Design review of the part built by this model. Coordinates are the model's own, in mm. Face numbers are marked on the shaded views. A direction names the side the tool comes from. Coordinates: 2 decimals unless noted, no trailing zeros. Order: outer loops, then holes, each group sorted by start corner. A loop starts at its lowest first (then second) coordinate and runs counter-clockwise, first axis right, second up. Notation, with made-up numbers: M -11.75,-31.75 L 30.25,-31.75 A17 cw 30.25,-6.75 Z; hole C -13,-12.75 d8. An arc over 180 degrees is marked long. Answer as a JSON object with one key per item and string values.
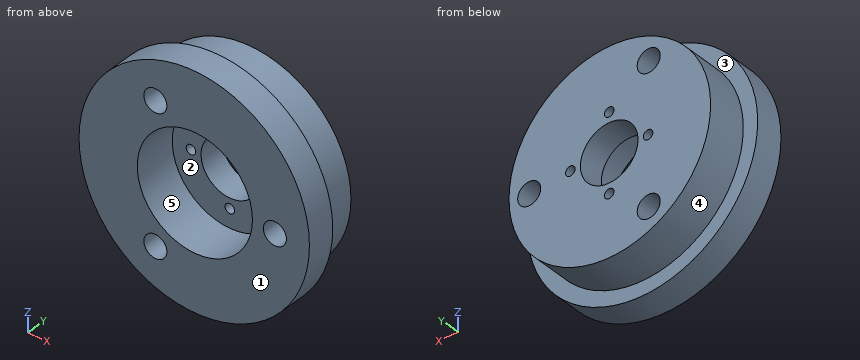
from build123d import *

# Parameters (mm, degrees)
SKETCH2_R               = 10
SKETCH2_R_2             = 1.65
CUT_EXTRUDE2_DEPTH      = 1
CUT_EXTRUDE2_DEPTH_BACK = 25
SKETCH2_5_R             = 20
SKETCH2_5_R_2           = 1.65
SKETCH2_5_R_3           = 10
CUT_EXTRUDE3_DEPTH      = 15
SKETCH3_R               = 4
CUT_EXTRUDE4_DEPTH      = 1
CUT_EXTRUDE4_DEPTH_BACK = 25


with BuildPart() as part:
    # Sketch1 → Revolve1 (revolve)
    with BuildSketch(Plane.XY):
        Polygon((-40, 10), (-35, 10), (-35, 24), (0, 24), (0, 0), (-40, 0), align=None)
    revolve(axis=Axis((0, -1000, 0), (0, 1, 0)))

    # Sketch2 → Cut-Extrude2 (cut, two sides)
    with BuildSketch(Plane.XZ) as cut_extrude2_sk:
        with Locations((0.220332098, -0.275415123)):
            Circle(SKETCH2_R)
        with Locations((13.720332098, -0.275415123)):
            Circle(SKETCH2_R_2)
        with Locations((0.220332098, -13.775415123)):
            Circle(SKETCH2_R_2)
        with Locations((-13.279667902, -0.275415123)):
            Circle(SKETCH2_R_2)
        with Locations((0.220332098, 13.224584877)):
            Circle(SKETCH2_R_2)
    extrude(amount=CUT_EXTRUDE2_DEPTH, mode=Mode.SUBTRACT)
    extrude(cut_extrude2_sk.sketch, amount=-CUT_EXTRUDE2_DEPTH_BACK, mode=Mode.SUBTRACT)

    # Sketch2<5> → Cut-Extrude3 (cut)
    with BuildSketch(Plane.XZ):
        with Locations((0.220332098, -0.275415123)):
            Circle(SKETCH2_5_R)
        with Locations((0.220332098, -13.775415123)):
            Circle(SKETCH2_5_R_2, mode=Mode.SUBTRACT)
        with Locations((13.720332098, -0.275415123)):
            Circle(SKETCH2_5_R_2, mode=Mode.SUBTRACT)
        with Locations((0.220332098, -0.275415123)):
            Circle(SKETCH2_5_R_3, mode=Mode.SUBTRACT)
        with Locations((-13.279667902, -0.275415123)):
            Circle(SKETCH2_5_R_2, mode=Mode.SUBTRACT)
        with Locations((0.220332098, 13.224584877)):
            Circle(SKETCH2_5_R_2, mode=Mode.SUBTRACT)
    extrude(amount=-CUT_EXTRUDE3_DEPTH, mode=Mode.SUBTRACT)

    # Sketch3 → Cut-Extrude4 (cut, two sides)
    with BuildSketch(Plane(origin=(0, 24, 0), x_dir=(1, 0, 0), z_dir=(0, 1, 0))) as cut_extrude4_sk:
        with Locations((28, 1.382050236)):
            Circle(SKETCH3_R)
        with Locations((-13.5, -24.11)):
            Circle(SKETCH3_R)
        with Locations((-13.5, 24.11473671)):
            Circle(SKETCH3_R)
    extrude(amount=CUT_EXTRUDE4_DEPTH, mode=Mode.SUBTRACT)
    extrude(cut_extrude4_sk.sketch, amount=-CUT_EXTRUDE4_DEPTH_BACK, mode=Mode.SUBTRACT)


solid = part.part
1) Tool access review of the marked faces 1 and 2: name each direction out of +Z, -Z, +X, -X, +Y, -Y from which nothing blocks a thin tool from reaching the whole face with its end or side.
Taken from the geometry:
{"face 1": "+Z, -Z, +X, -X, -Y", "face 2": "-Y"}
2) Add section D-D (x = 21.5). State the section outline as (y, z) points, and give its area (3 significant figures).
Taken from the geometry:
{"outline": "M 0,-33.73 L 10,-33.73 L 10,-27.62 L 24,-27.62 L 24,27.62 L 10,27.62 L 10,33.73 L 0,33.73 Z", "area": "1,450 mm2"}
3) Add section C-C (y = 17.25). Count the separate pieces of the cut face and the enclosed holes in it, and give its area (3 significant figures).
Taken from the geometry:
{"separate pieces": "1", "enclosed holes": "8", "area": "3,350 mm2"}
4) Add section A-A (z = 27). State the section outline as (x, y) points, and give its area (3 significant figures).
Taken from the geometry:
{"outline": "M -29.51,0 L -16.27,0 L -16.27,24 L -22.27,24 L -22.27,10 L -29.51,10 Z; M -10.73,0 L 29.51,0 L 29.51,10 L 22.27,10 L 22.27,24 L -10.73,24 Z", "area": "1,080 mm2"}
5) Mouldability with a two-part tool opening along X and no side actions: class the marked faces 3, 4 and 5 as released by +X, released by -X, zero draft, split by the parting line, or undercut.
Taken from the geometry:
{"face 3": "zero draft", "face 4": "split by the parting line", "face 5": "undercut"}
6) Add section B-B (x = 4). State the section outline as (y, z) points.
Taken from the geometry:
{"outline": "M 0,-39.8 L 10,-39.8 L 10,-34.77 L 24,-34.77 L 24,-9.53 L 15,-9.53 L 15,-19.92 L 0,-19.92 Z; M 0,19.36 L 15,19.36 L 15,8.98 L 24,8.98 L 24,34.77 L 10,34.77 L 10,39.8 L 0,39.8 Z"}
7) Insertion check: pin 1 Ø4 at (x, z) = (0.22, -13.78) entering from -Y; pin 2 Ø2 at (x, z) = (13.72, -0.28) entering from -Y; pin 3 Ø12 at (x, y) = (18, 11) entering from +Z; pin 4 Ø4 at (y, z) = (13, -16) entering from -X. Each pin has a flat end and moves straight along its axis. Give the tip position at first contact, or say it passes through.
Taken from the geometry:
{"pin 1": "stops at y = 15", "pin 2": "passes through", "pin 3": "stops at z = 38.13", "pin 4": "stops at x = -32.08"}
8) To check wall thickness, follow L1, parallel to Z at x = -13.5, y = 13.25; L2, parallel to X at y = 20, z = -13; L3, parallel to X at y = 3, z = 24. State the ranges of each line that lie inside material, in increasing order.
Taken from the geometry:
{"L1": "z = -32.29 to -28.11, -20.11 to -14.83, 14.28 to 20.11, 28.11 to 32.29", "L2": "x = -32.5 to -1.24, 1.68 to 32.5", "L3": "x = -32 to -17.5, -9.5 to 32"}
